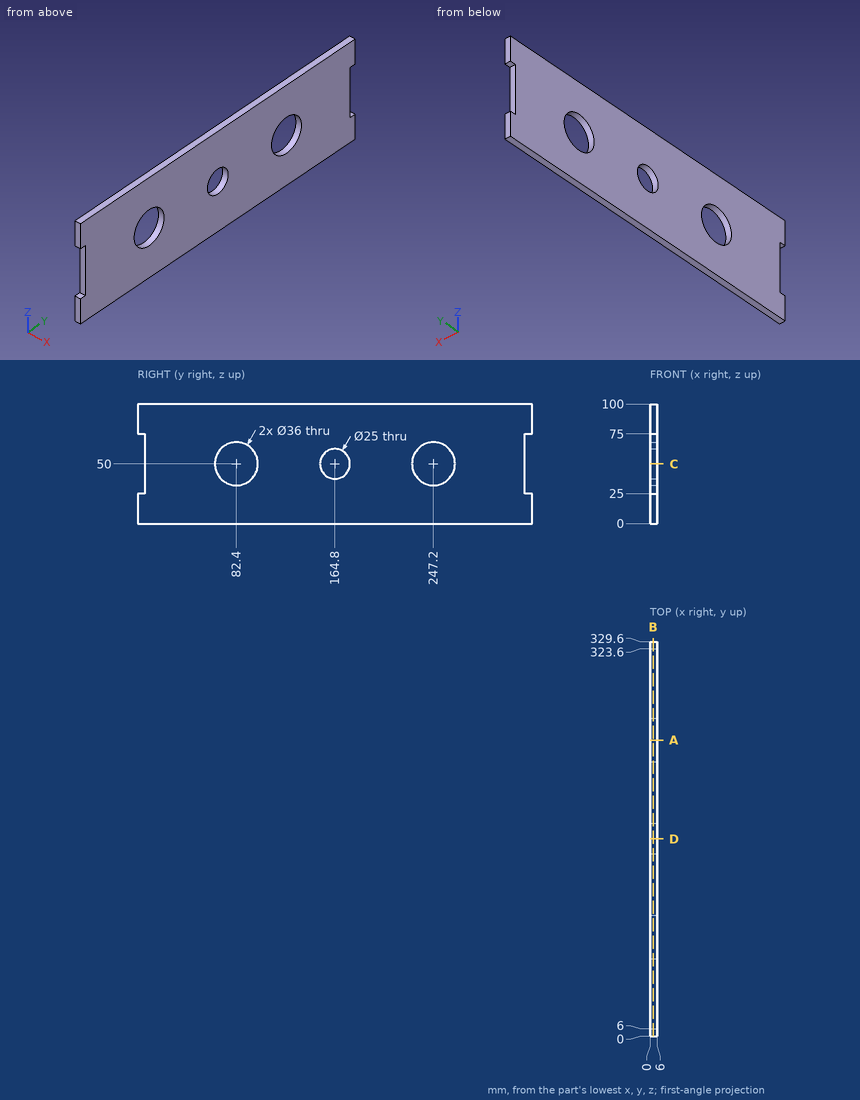
Answer from the drawing. Dimensions are ordinates in mm from the lowest x, y and z of the part. Give positions to 0.01 mm unless a question says otherwise; leave off trailing zeros. Order: outer loops, then holes, each group sorted by start corner. A loop starts at its lowest first (then second) coordinate and runs counter-clockwise, first axis right, second up.
Item 1: Find the intervals of material crossed by probe 1 along Y at (x, z) = (1.1, 49); probe 2 along Y at (x, z) = (3.6, 43.5); probe 3 along Z at (x, y) = (2.1, 164.5), in increasing order.
From the geometry:
probe 1: y = 6 to 64.43, 100.37 to 152.34, 177.26 to 229.23, 265.17 to 323.6
probe 2: y = 6 to 65.61, 99.19 to 154.12, 175.48 to 230.41, 263.99 to 323.6
probe 3: z = 0 to 37.5, 62.5 to 100
Item 2: The part is cut by section C-C, the plane z = 50. Give the vertices of the cut face in (x, y).
From the geometry:
outline: (0, 6) - (6, 6) - (6, 64.4) - (0, 64.4) - close; (0, 100.4) - (6, 100.4) - (6, 152.3) - (0, 152.3) - close; (0, 177.3) - (6, 177.3) - (6, 229.2) - (0, 229.2) - close; (0, 265.2) - (6, 265.2) - (6, 323.6) - (0, 323.6) - close
Item 3: Given pin 1 Ø1 at (x, z) = (2.5, 56.5) entering from -Y; pin 2 Ø1.8 at (x, z) = (2.5, 48) entering from +Y, each flat-ended and moving along its own axis, determine where each tip first touches the part or whether it passes through.
From the geometry:
pin 1: stops at y = 6
pin 2: stops at y = 323.6
Item 4: The part is cut by section B-B, the plane x = 2.6. Give the vertices of the cut face in (y, z).
From the geometry:
outline: (0, 0) - (329.6, 0) - (329.6, 25) - (323.6, 25) - (323.6, 75) - (329.6, 75) - (329.6, 100) - (0, 100) - (0, 75) - (6, 75) - (6, 25) - (0, 25) - close; hole circle Ø36 at (82.4, 50); hole circle Ø25 at (164.8, 50); hole circle Ø36 at (247.2, 50)
Item 5: The part is cut by section A-A, the plane y = 247.2. Give the vertices of the cut face in (x, z), and give its area (3 significant figures).
From the geometry:
outline: (0, 0) - (6, 0) - (6, 32) - (0, 32) - close; (0, 68) - (6, 68) - (6, 100) - (0, 100) - close
area: 384 mm2
Item 6: The part is cut by section D-D, the plane y = 164.8. Give the vertices of the cut face in (x, z), and give its area (3 significant figures).
From the geometry:
outline: (0, 0) - (6, 0) - (6, 37.5) - (0, 37.5) - close; (0, 62.5) - (6, 62.5) - (6, 100) - (0, 100) - close
area: 450 mm2
